The listing builds one solid part. Answer for the finished solid, in the listing's coordinates (mm). A direction names the side the tool comes from. Give positions to 0.01 mm unless a question says otherwise; leave off trailing zeros. Write each loop counter-clockwise with the first axis right and the second up, starting at its lowest first coordinate (ties: lowest second). Pieces come first, ordered by that corner, then holes. Notation, with made-up numbers: M -13,-22.5 L 35,-22.5 A21 ccw 35,-3.5 Z; hole C 46,40.5 d6. An arc over 180 degrees is marked long. Answer as a JSON object with one key per item and string values.
```python
from build123d import *

# Parameters (mm, degrees)
F0_W     = 444.5
F0_H     = 304.8
F1_DEPTH = 21.971
F2_W     = 431.8
F2_H     = 292.1
F3_DEPTH = 5.715
F5_W     = 393.7
F5_H     = 254
F6_DEPTH = 27.687
F9_D     = 3.7973


with BuildPart() as f1:
    # F0 (on Top) → F1 (new body)
    with BuildSketch(Plane.XY):
        with Locations((222.25, 152.4)):
            Rectangle(F0_W, F0_H)
    extrude(amount=F1_DEPTH)

    # F2 (on face) → F3 (join)
    with BuildSketch(Plane(origin=(0, 0, 0), x_dir=(1, 0, 0), z_dir=(0, 0, -1))):
        with Locations((222.25, -152.4)):
            Rectangle(F2_W, F2_H)
    extrude(amount=F3_DEPTH)

    # F5 (on face) → F6 (cut, through all)
    with BuildSketch(Plane.XY.offset(21.971)):
        with Locations((222.25, 152.4)):
            Rectangle(F5_W, F5_H)
    extrude(amount=-F6_DEPTH, mode=Mode.SUBTRACT)

    # F9 (through all)
    with Locations(Plane.XY.offset(21.971)):
        with Locations((429.26, 254), (429.26, 215.9), (429.26, 88.9), (429.26, 50.8)):
            Hole(F9_D / 2)


solid = f1.part
```
1. The mould has two halves that part along X. Classify faces 3 (the flat face through (221, 282, -5.715)), 4 (the flat face through (25.4, 151, 8)), 5 (the flat face through (444.5, 150, 11)), 6 (the flat face through (419.1, 151, 8)): released by +X, released by -X, zero draft, split by the parting line, or undercut.
Verdict:
{"face 3": "zero draft", "face 4": "undercut", "face 5": "released by +X", "face 6": "undercut"}
2. Consider line 1 along X through (y, z) = (254, 4.25); line 2 along Y through (x, z) = (429.26, 13.5); line 3 along Y through (x, z) = (225.5, 19). Determine where each line is inside the solid, lowest interval first.
Verdict:
{"line 1": "x = 0 to 25.4, 419.1 to 427.36, 431.16 to 444.5", "line 2": "y = 0 to 48.9, 52.7 to 87, 90.8 to 214, 217.8 to 252.1, 255.9 to 304.8", "line 3": "y = 0 to 25.4, 279.4 to 304.8"}
3. Flat-ended cylindrical pins translate along their axes: pin 1 (6 mm diameter, centred on x = 429.26, y = 50.8, fed in from -Z) (3 decimals); pin 2 (4.5 mm diameter, centred on x = 273, z = -2.5, fed in from -Y); pin 3 (2.5 mm diameter, centred on x = 429.26, y = 88.9, fed in from -Z); pin 4 (6.5 mm diameter, centred on y = 89.5, z = -4, fed in from +X). Find the tip coordinate at first contact, or state that the pin passes through.
Verdict:
{"pin 1": "stops at z = -5.715", "pin 2": "stops at y = 6.35", "pin 3": "passes through", "pin 4": "stops at x = 438.15"}
4. A cutting plane is placed at A-A, the plane x = 111. Give the vertices of the cut face in (y, z) (3 decimals), plus the area to 3 significant figures.
Verdict:
{"outline": "M 0,0 L 6.35,0 L 6.35,-5.715 L 25.4,-5.715 L 25.4,21.971 L 0,21.971 Z; M 279.4,-5.715 L 298.45,-5.715 L 298.45,0 L 304.8,0 L 304.8,21.971 L 279.4,21.971 Z", "area": "1,330 mm2"}
5. For faces 1 (the flat face through (219, 304.8, 11)), 2 (the flat face through (219, 25.4, 8)), determine the directions among +Z, -Z, +X, -X, +Y, -Y from which every point of the face is accessible in a straight line to the end or side of a thin tool.
Verdict:
{"face 1": "+Z, -Z, +X, -X, +Y", "face 2": "+Z, -Z"}
6. A cutting plane is placed at C-C, the plane z = 12.25. Give the vertices of the cut face in (x, y).
Verdict:
{"outline": "M 0,0 L 444.5,0 L 444.5,304.8 L 0,304.8 Z; hole M 25.4,25.4 L 419.1,25.4 L 419.1,279.4 L 25.4,279.4 Z; hole C 429.26,50.8 d3.8; hole C 429.26,88.9 d3.8; hole C 429.26,215.9 d3.8; hole C 429.26,254 d3.8"}
7. A cutting plane is placed at B-B, the plane y = 34.5. Give the vertices of the cut face in (x, z) (3 decimals), plus the area to 3 significant figures.
Verdict:
{"outline": "M 0,0 L 6.35,0 L 6.35,-5.715 L 25.4,-5.715 L 25.4,21.971 L 0,21.971 Z; M 419.1,-5.715 L 438.15,-5.715 L 438.15,0 L 444.5,0 L 444.5,21.971 L 419.1,21.971 Z", "area": "1,330 mm2"}
